Can you work these out from the drawing? Everything is in mm from the part's minimum corner. A direction names the side the tool comes from. Round coordinates to 2 decimals unless told otherwise and drop trailing zeros. Loops run counter-clockwise (first coordinate to the right, second up) from the corner with the lowest first, then second, coordinate; pieces in that order, holes last. Notation, with made-up numbers: (83, -16.75) -> (103, -16.75) arc R30 ccw to (103, 10.25) -> close; hole circle Ø9 at (60.5, 88). An arc over 180 degrees is marked (long way). Answer as a JSON object with one key per item and string values.
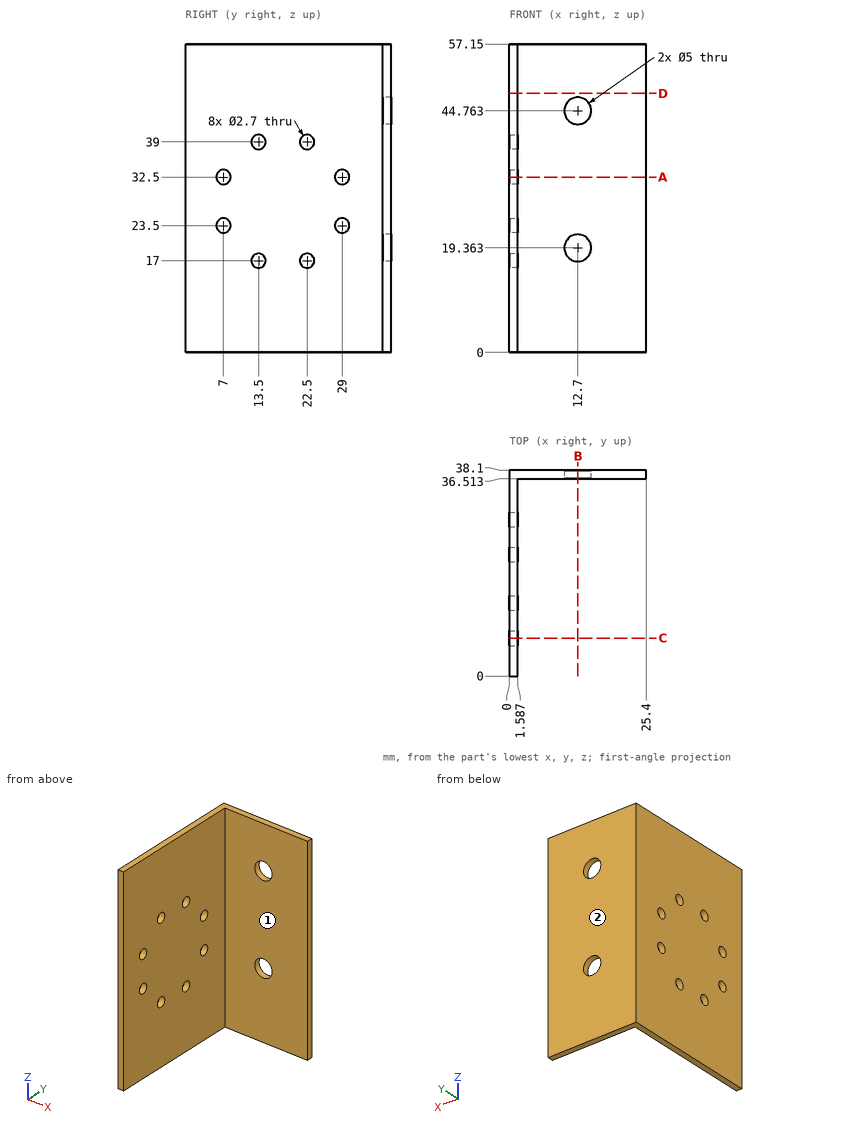
Q1. If I drill on L1, parallel to Y at x = 1.05, z = 17; L2, parallel to Y at x = 0.75, z = 32.5; L3, parallel to Y at x = 2.75, z = 27, over which ranges is the centre line in solid material (lowest first)? Write a range as [from, to].
Determined:
{"L1": "[0, 12.15], [14.85, 21.15], [23.85, 38.1]", "L2": "[0, 5.65], [8.35, 27.65], [30.35, 38.1]", "L3": "[36.51, 38.1]"}
Q2. On a 3-axis mill with a long thin cutter (end or side, diameter ignored), from which of +Z, -Z, +X, -X, +Y, -Y can I reach the whole of each face in a straight line? I mean the marked faces 1 and 2. Say none if no direction works.
Determined:
{"face 1": "+Z, -Z, +X, -Y", "face 2": "+Z, -Z, +X, -X, +Y"}
Q3. I'm going to push flat-ended pins straight in: pin 1 (1.6 mm diameter, centred on y = 29, z = 23.5, fed in from -X); pin 2 (3 mm diameter, centred on y = 7, z = 32.5, fed in from +X); pin 3 (6 mm diameter, centred on x = 16.5, z = 51, fed in from -Y). Where does each tip first touch, or does it pass through?
Determined:
{"pin 1": "through", "pin 2": "x = 1.59", "pin 3": "y = 36.51"}
Q4. I want a section at B-B, the plane x = 12.7. Write out the boundary of the cut face in (y, z).
Determined:
{"outline": "(36.51, 0) -> (38.1, 0) -> (38.1, 16.86) -> (36.51, 16.86) -> close; (36.51, 21.86) -> (38.1, 21.86) -> (38.1, 42.26) -> (36.51, 42.26) -> close; (36.51, 47.26) -> (38.1, 47.26) -> (38.1, 57.15) -> (36.51, 57.15) -> close"}
Q5. I want a section at D-D, the plane z = 48. Write out the boundary of the cut face in (x, y).
Determined:
{"outline": "(0, 0) -> (1.59, 0) -> (1.59, 36.51) -> (25.4, 36.51) -> (25.4, 38.1) -> (0, 38.1) -> close"}
Q6. I want a section at A-A, the plane z = 32.5. Write out the boundary of the cut face in (x, y).
Determined:
{"outline": "(0, 0) -> (1.59, 0) -> (1.59, 5.65) -> (0, 5.65) -> close; (0, 8.35) -> (1.59, 8.35) -> (1.59, 27.65) -> (0, 27.65) -> close; (0, 30.35) -> (1.59, 30.35) -> (1.59, 36.51) -> (25.4, 36.51) -> (25.4, 38.1) -> (0, 38.1) -> close"}
Q7. I want a section at C-C, the plane y = 7. Write out the boundary of the cut face in (x, z).
Determined:
{"outline": "(0, 0) -> (1.59, 0) -> (1.59, 22.15) -> (0, 22.15) -> close; (0, 24.85) -> (1.59, 24.85) -> (1.59, 31.15) -> (0, 31.15) -> close; (0, 33.85) -> (1.59, 33.85) -> (1.59, 57.15) -> (0, 57.15) -> close"}
